```python
from build123d import *

# Parameters (mm, degrees)
SKETCH_1_R          = 57.5
SKETCH_1_R_2        = 22
EXTRUDE_1_DEPTH     = 3
SKETCH_2_W          = 140.517246729
SKETCH_2_H          = 54.837850232
SKETCH_2_H_2        = 57.45712313
CUT_EXTRUDE_1_DEPTH = 82.372599811
SKETCH_3_W          = 35
SKETCH_3_H          = 9.6
CUT_EXTRUDE_2_DEPTH = 0.15


with BuildPart() as part:
    # Эскиз1 → Бобышка-Вытянуть1 (new body)
    with BuildSketch(Plane.XY):
        Circle(SKETCH_1_R)
        Circle(SKETCH_1_R_2, mode=Mode.SUBTRACT)
    extrude(amount=EXTRUDE_1_DEPTH)

    # Эскиз2 → Вырез-Вытянуть1 (cut, through all)
    with BuildSketch(Plane.XY.offset(3)):
        with Locations((-1.418485275, 64.418925116)):
            Rectangle(SKETCH_2_W, SKETCH_2_H)
        with Locations((-1.418485275, -65.728561565)):
            Rectangle(SKETCH_2_W, SKETCH_2_H_2)
    extrude(amount=-CUT_EXTRUDE_1_DEPTH, mode=Mode.SUBTRACT)

    # Эскиз3 → Вырез-Вытянуть2 (cut)
    with BuildSketch(Plane.XY.offset(3)):
        Polygon((-1.5, 37), (1.5, 37), (1.5, 7.8), (63.743793757, 7.8), (63.743793757, 4.8), (1.5, 4.8), (1.5, -4.8), (65.582153435, -4.8), (65.582153435, -7.8), (1.5, -7.8), (1.5, -37), (-1.5, -37), (-1.5, -7.8), (-73.634100968, -7.8), (-73.634100968, -4.8), (-41, -4.8), (-41, 4.8), (-72.371033765, 4.8), (-72.371033765, 7.8), (-1.5, 7.8), align=None)
        with Locations((-19, 0)):
            Rectangle(SKETCH_3_W, SKETCH_3_H, mode=Mode.SUBTRACT)
    extrude(amount=-CUT_EXTRUDE_2_DEPTH, mode=Mode.SUBTRACT)


solid = part.part
```
Here's how the part is built. I have some questions about the finished solid (model axes, mm). A direction names the side the tool comes from. Coordinates: 2 decimals unless noted, no trailing zeros. Write each loop counter-clockwise with the first axis right and the second up, starting at its lowest first coordinate (ties: lowest second). Pieces come first, ordered by that corner, then holes. Notation, with made-up numbers: (-40, -33) - (-15, -33) arc R15 cw to (-15, -21) - close; hole circle Ø3 at (-30.75, 48.25). An arc over 180 degrees is marked (long way). One line per item, written item: value.
1) Suppose I cut it at D-D on x = 46.5. Write out the boundary of the cut face in (y, z).
Model answer:
outline: (-33.82, 0) - (33.82, 0) - (33.82, 3) - (7.8, 3) - (7.8, 2.85) - (4.8, 2.85) - (4.8, 3) - (-4.8, 3) - (-4.8, 2.85) - (-7.8, 2.85) - (-7.8, 3) - (-33.82, 3) - close
2) Suppose I cut it at A-A on x = 0. Write out the boundary of the cut face in (y, z).
Model answer:
outline: (-37, 0) - (-22, 0) - (-22, 2.85) - (-37, 2.85) - close; (22, 0) - (37, 0) - (37, 2.85) - (22, 2.85) - close
3) I'm going to push flat-ended pins straight in: P1, Ø1.5, axis at y = 11.5, z = 1.5, coming from the +X side; P2, Ø1, axis at y = -9, z = 2.5, coming from the +X side. Where does each tip first touch, or does it pass through?
Model answer:
P1: stops at x = 56.49
P2: stops at x = 56.87
4) On a 3-axis mill with a long thin cutter (end or side, diameter ignored), from which of +Z, -Z, +X, -X, +Y, -Y can I reach the whole of each face in a straight line? I mean faces 1 (the flat face through (0, -29, 2.85)), 2 (the flat face through (39, -6, 2.85)), 3 (the cylindrical face through (-4.769, -21.477, 1.479)). Say none if no direction works.
Model answer:
face 1: +Z, +Y, -Y
face 2: +Z, +X, -X
face 3: +Z, -Z
5) Suppose I cut it at C-C on z = 0.55. Write out the boundary of the cut face in (x, y), and give its area (3 significant figures).
Model answer:
outline: (-44.01, -37) - (44.01, -37) arc R57.5 ccw to (44.01, 37) - (-44.01, 37) arc R57.5 ccw to start; hole circle Ø44 at (0, 0)
area: 6,360 mm²
6) I need wall thicknesses on line 1 along Y through (x, z) = (29, 2.95); line 2 along Y through (x, z) = (0, 0.95); line 3 along X through (y, z) = (0.5, 1.15). Which ranges of each line are inside material? Lowest first, please.
Model answer:
line 1: y = -37 to -7.8, -4.8 to 4.8, 7.8 to 37
line 2: y = -37 to -22, 22 to 37
line 3: x = -57.5 to -21.99, 21.99 to 57.5
7) We'd pull the mould along Y, two halves only. Please class faces 4 (the flat face through (39, 6, 2.85)), 5 (the cylindrical face through (57.497, -0.563, 1.479)), 6 (the flat face through (-1, -24, 0)): pulls with the +Y half, pulls with the -Y half, needs draft (parallel to the pull), parting line crosses it, or undercut.
Model answer:
face 4: undercut
face 5: parting line crosses it
face 6: needs draft
8) Suppose I cut it at B-B on y = 0. Write out the boundary of the cut face in (x, z).
Model answer:
outline: (-57.5, 0) - (-22, 0) - (-22, 3) - (-36.5, 3) - (-36.5, 2.85) - (-41, 2.85) - (-41, 3) - (-57.5, 3) - close; (22, 0) - (57.5, 0) - (57.5, 3) - (22, 3) - close
